from build123d import *

# Parameters (mm, degrees)
SKETCH_2_R          = 9
EXTRUDE_1_DEPTH     = 65
CUT_EXTRUDE_START   = 9
CUT_EXTRUDE_1_DEPTH = 5
CUT_EXTRUDE_2_DEPTH = 5


with BuildPart() as part:
    # 草图2 → 凸台-拉伸1 (new body)
    with BuildSketch(Plane(origin=(0, 10, 0), x_dir=(1, 0, 0), z_dir=(0, 1, 0))):
        with Locations(Location((0, 0, 0), (0, 0, 270))):
            Circle(SKETCH_2_R)
    extrude(amount=EXTRUDE_1_DEPTH)

    # 草图4 → 切除-拉伸1 (cut)
    with BuildSketch(Plane.XY.offset(CUT_EXTRUDE_START)):
        with BuildLine():
            Line((-3.441616095, 27.248377589), (-3.441616095, 39.696776231))
            ThreePointArc((-3.441616095, 39.696776231), (0, 43.138392326), (3.441616095, 39.696776231))
            Line((3.441616095, 39.696776231), (3.441616095, 27.248377589))
            ThreePointArc((3.441616095, 27.248377589), (0, 23.806761494), (-3.441616095, 27.248377589))
        make_face()
    extrude(amount=-CUT_EXTRUDE_1_DEPTH, mode=Mode.SUBTRACT)

    # 草图5 → 切除-拉伸2 (cut)
    with BuildSketch(Plane.XY.offset(9)):
        with BuildLine():
            Line((-3.590752792, 51.789816315), (-3.590752792, 64.069272059))
            ThreePointArc((-3.590752792, 64.069272059), (0, 67.660024851), (3.590752792, 64.069272059))
            Line((3.590752792, 64.069272059), (3.590752792, 51.789816315))
            ThreePointArc((3.590752792, 51.789816315), (0, 48.199063523), (-3.590752792, 51.789816315))
        make_face()
    extrude(amount=-CUT_EXTRUDE_2_DEPTH, mode=Mode.SUBTRACT)


solid = part.part
Geometry check sheet. Reference: the model listing, model coordinates, mm. A direction names the side the tool comes from. Give positions to 0.01 mm unless a question says otherwise; leave off trailing zeros. Loops run counter-clockwise (first coordinate to the right, second up) from the corner with the lowest first, then second, coordinate; pieces in that order, holes last. Notation, with made-up numbers: (-1.5, 4) -> (19.5, 4) arc R14 ccw to (19.5, 27) -> close; hole circle Ø9 at (-22, 9.5). An arc over 180 degrees is marked (long way). Answer in a Markdown table with one row per item. Add a question column.
1) Set-up check for faces 1 (the face through (0.1, 48.2, 6.5)), 2 (the face through (0, 42, -9)): record each of +Z, -Z, +X, -X, +Y, -Y from which the full face is reachable in a straight line by a thin tool's end or side.
2) Cross-section at D-D on x = -2.5. Record the boundary of the cut face in (y, z).
3) Draft check along Y on faces 3 (the face through (0, 10, 0)), 4 (the face through (-3.591, 58, 6)), 5 (the face through (0, 75, 0)). Enter one of: pulls with the +Y half, pulls with the -Y half, needs draft (parallel to the pull), parting line crosses it, or undercut.
4) Gauge pin test, flat ends, axial feed: P1, Ø1.3, axis at y = 60.5, z = 5.5, coming from the -X side; P2, Ø2, axis at x = -0.5, y = 30, coming from the +Z side; P3, Ø3, axis at y = 43, z = -5.5, coming from the -X side. Record the tip position at first contact, or that the pin passes through.
5) Cross-section at A-A on x = 0. Record the boundary of the cut face in (y, z).
6) Cross-section at B-B on y = 30. Record the boundary of the cut face in (x, z).
7) Material ranges on probe 1 along Y at (x, z) = (0.5, 5); probe 2 along X at (y, z) = (34.5, 6.5); probe 3 along Y at (x, z) = (-2.75, 8), recorded low to high. Write a range as from..to.
8) Cross-section at C-C on z = -7.25. Record the boundary of the cut face in (x, y).
Outcome:
| question | item | result |
|---|---|---|
| 1 | face 1 | +Z |
| 1 | face 2 | +Y, -Y |
| 2 | outline | (10, -8.65) -> (75, -8.65) -> (75, 8.65) -> (66.65, 8.65) -> (66.65, 4) -> (49.21, 4) -> (49.21, 8.65) -> (42.06, 8.65) -> (42.06, 4) -> (24.88, 4) -> (24.88, 8.65) -> (10, 8.65) -> close |
| 3 | face 3 | pulls with the -Y half |
| 3 | face 4 | undercut |
| 3 | face 5 | pulls with the +Y half |
| 4 | P1 | stops at x = -7.58 |
| 4 | P2 | stops at z = 4 |
| 4 | P3 | stops at x = -8.06 |
| 5 | outline | (10, -9) -> (75, -9) -> (75, 9) -> (67.66, 9) -> (67.66, 4) -> (48.2, 4) -> (48.2, 9) -> (43.14, 9) -> (43.14, 4) -> (23.81, 4) -> (23.81, 9) -> (10, 9) -> close |
| 6 | outline | (-3.44, 4) -> (-3.44, 8.32) arc R9 ccw (long way) to (3.44, 8.32) -> (3.44, 4) -> close |
| 7 | probe 1 | y = 10..23.84, 43.1..48.23, 67.63..75 |
| 7 | probe 2 | x = -6.22..-3.44, 3.44..6.22 |
| 7 | probe 3 | y = 10..25.18, 41.77..49.48, 66.38..75 |
| 8 | outline | (-5.33, 10) -> (5.33, 10) -> (5.33, 75) -> (-5.33, 75) -> close |
